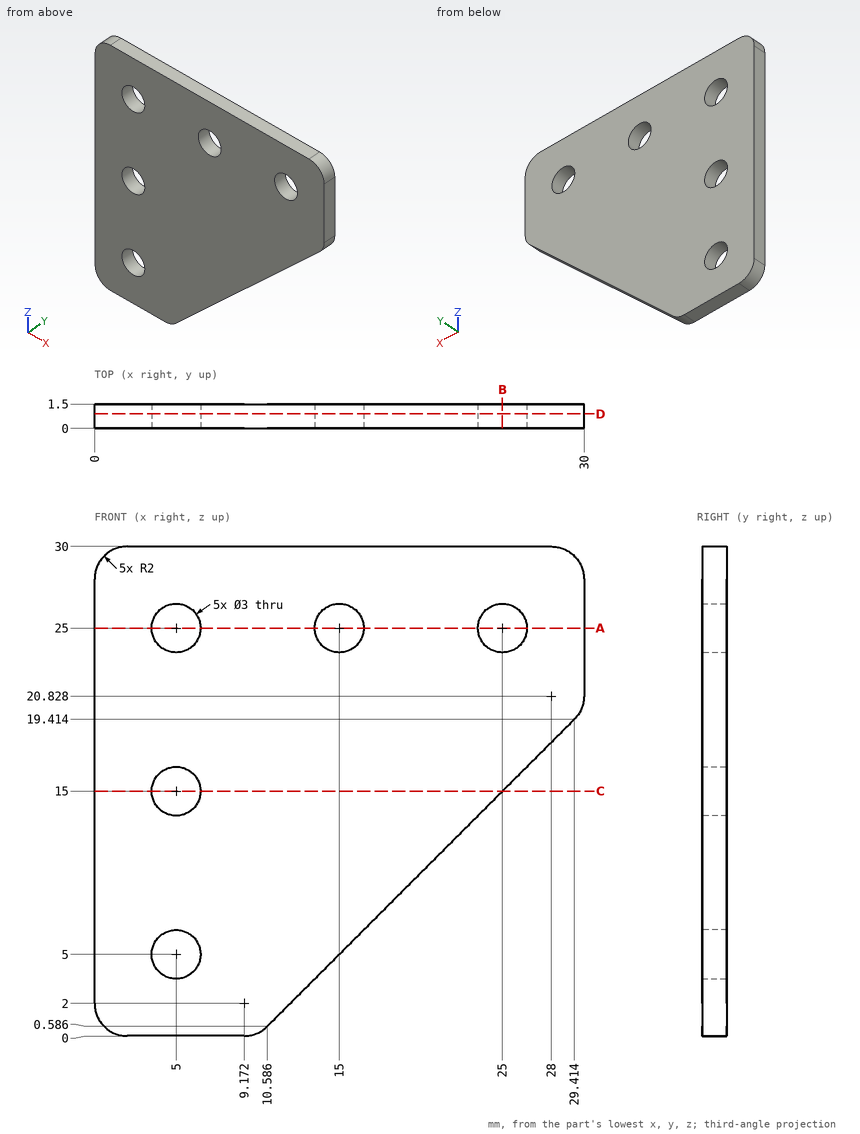
The drawing under review shows one solid part. Ordinate dimensions are in mm from its lowest x, y, z. Coordinates: 2 decimals unless noted, no trailing zeros. Order: outer loops, then holes, each group sorted by start corner. A loop starts at its lowest first (then second) coordinate and runs counter-clockwise, first axis right, second up. Notation, with made-up numbers: (38, 79.25) - (46, 79.25) arc R19 ccw to (46, 91.25) - close; hole circle Ø4 at (88, 65.25). An arc over 180 degrees is marked (long way). Put each result on its own line as item: value.
1) Take a section at D-D, the plane y = 0.9. Give the boundary of the cut face in (x, z) (1 decimal), and give its area (3 significant figures).
Response values:
outline: (0, 2) arc R2 ccw to (2, 0) - (9.2, 0) arc R2 ccw to (10.6, 0.6) - (29.4, 19.4) arc R2 ccw to (30, 20.8) - (30, 28) arc R2 ccw to (28, 30) - (2, 30) arc R2 ccw to (0, 28) - close; hole circle Ø3 at (5, 5); hole circle Ø3 at (5, 15); hole circle Ø3 at (5, 25); hole circle Ø3 at (15, 25); hole circle Ø3 at (25, 25)
area: 662 mm²
2) Wall thickness on L1, parallel to X at y = 0.35, z = 25; L2, parallel to X at y = 0.85, z = 24; L3, parallel to X at y = 1, z = 5: over which ranges is each line inside the solid? List them lowest first. Write a range as from..to.
Response values:
L1: x = 0..3.5, 6.5..13.5, 16.5..23.5, 26.5..30
L2: x = 0..3.88, 6.12..13.88, 16.12..23.88, 26.12..30
L3: x = 0..3.5, 6.5..15
3) Take a section at A-A, the plane z = 25. Give the boundary of the cut face in (x, y), and give its area (3 significant figures).
Response values:
outline: (0, 0) - (3.5, 0) - (3.5, 1.5) - (0, 1.5) - close; (6.5, 0) - (13.5, 0) - (13.5, 1.5) - (6.5, 1.5) - close; (16.5, 0) - (23.5, 0) - (23.5, 1.5) - (16.5, 1.5) - close; (26.5, 0) - (30, 0) - (30, 1.5) - (26.5, 1.5) - close
area: 31.5 mm²
4) Take a section at B-B, the plane x = 25. Give the boundary of the cut face in (y, z), and give its area (3 significant figures).
Response values:
outline: (0, 15) - (1.5, 15) - (1.5, 23.5) - (0, 23.5) - close; (0, 26.5) - (1.5, 26.5) - (1.5, 30) - (0, 30) - close
area: 18.0 mm²
5) Take a section at C-C, the plane z = 15. Give the boundary of the cut face in (x, y).
Response values:
outline: (0, 0) - (3.5, 0) - (3.5, 1.5) - (0, 1.5) - close; (6.5, 0) - (25, 0) - (25, 1.5) - (6.5, 1.5) - close
